```python
from build123d import *

# Parameters (mm, degrees)
AX_PCB_FLAT_FRONT_COMPARTMENT_START        = 25
SKETCH_1_W                                 = 90
SKETCH_1_H                                 = 130
SKETCH_1_R                                 = 1.75
AX_PCB_FLAT_FRONT_COMPARTMENT_DEPTH        = 1.6
J10_FRONT_CAMERA_HEADER_START              = 26.6
SKETCH_2_W                                 = 58.4
SKETCH_2_H                                 = 8.8
J10_FRONT_CAMERA_HEADER_DEPTH              = 8
J11_REAR_IDC40_START                       = 26.6
SKETCH_3_W                                 = 58.4
SKETCH_3_H                                 = 8.8
J11_REAR_IDC40_DEPTH                       = 8
HDMI_LEFT_START                            = 26.6
SKETCH_5_W                                 = 17
SKETCH_5_H                                 = 12
HDMI_LEFT_DEPTH                            = 8
USB_HOST_LEFT_START                        = 26.6
SKETCH_6_W                                 = 18
SKETCH_6_H                                 = 14
USB_HOST_LEFT_DEPTH                        = 12
RJ45_LEFT_START                            = 26.6
SKETCH_7_W                                 = 22
SKETCH_7_H                                 = 16
RJ45_LEFT_DEPTH                            = 14
DC5521_APPROX_BODY_CLEAR_CAMERA_EDGE_START = 26.6
SKETCH_8_W                                 = 12
SKETCH_8_H                                 = 12
DC5521_APPROX_BODY_CLEAR_CAMERA_EDGE_DEPTH = 12


with BuildPart() as part:
    # 草图1 → AX_PCB_flat_front_compartment (new body)
    with BuildSketch(Plane.XY.offset(AX_PCB_FLAT_FRONT_COMPARTMENT_START)):
        with Locations((0, -77)):
            Rectangle(SKETCH_1_W, SKETCH_1_H)
        with Locations((-41, -138)):
            Circle(SKETCH_1_R, mode=Mode.SUBTRACT)
        with Locations((41, -138)):
            Circle(SKETCH_1_R, mode=Mode.SUBTRACT)
        with Locations((41, -16)):
            Circle(SKETCH_1_R, mode=Mode.SUBTRACT)
        with Locations((-41, -16)):
            Circle(SKETCH_1_R, mode=Mode.SUBTRACT)
    extrude(amount=AX_PCB_FLAT_FRONT_COMPARTMENT_DEPTH)

    # 草图2 → J10_front_camera_header (add)
    with BuildSketch(Plane.XY.offset(J10_FRONT_CAMERA_HEADER_START)):
        with Locations((0, -137.5)):
            Rectangle(SKETCH_2_W, SKETCH_2_H)
    extrude(amount=J10_FRONT_CAMERA_HEADER_DEPTH)

    # 草图3 → J11_rear_IDC40 (add)
    with BuildSketch(Plane.XY.offset(J11_REAR_IDC40_START)):
        with Locations((0, -16.5)):
            Rectangle(SKETCH_3_W, SKETCH_3_H)
    extrude(amount=J11_REAR_IDC40_DEPTH)

    # 草图5 → HDMI_left (add)
    with BuildSketch(Plane.XY.offset(HDMI_LEFT_START)):
        with Locations((-39.5, -37)):
            Rectangle(SKETCH_5_W, SKETCH_5_H)
    extrude(amount=HDMI_LEFT_DEPTH)

    # 草图6 → USB_HOST_left (add)
    with BuildSketch(Plane.XY.offset(USB_HOST_LEFT_START)):
        with Locations((-39, -97)):
            Rectangle(SKETCH_6_W, SKETCH_6_H)
    extrude(amount=USB_HOST_LEFT_DEPTH)

    # 草图7 → RJ45_left (add)
    with BuildSketch(Plane.XY.offset(RJ45_LEFT_START)):
        with Locations((-37, -60)):
            Rectangle(SKETCH_7_W, SKETCH_7_H)
    extrude(amount=RJ45_LEFT_DEPTH)

    # 草图8 → DC5521_approx_body_clear_camera_edge (add)
    with BuildSketch(Plane.XY.offset(DC5521_APPROX_BODY_CLEAR_CAMERA_EDGE_START)):
        with Locations((-42, -128)):
            Rectangle(SKETCH_8_W, SKETCH_8_H)
    extrude(amount=DC5521_APPROX_BODY_CLEAR_CAMERA_EDGE_DEPTH)


solid = part.part
```
Verification items for the finished model (mm, model axes). A direction names the side the tool comes from. Coordinates: 2 decimals unless noted, no trailing zeros. Write each loop counter-clockwise with the first axis right and the second up, starting at its lowest first coordinate (ties: lowest second). Pieces come first, ordered by that corner, then holes. Notation, with made-up numbers: M 32,45 L 62,45 A32 ccw 62,79 Z; hole C -6.75,41 d4. An arc over 180 degrees is marked long. One line per item, written item: value.
Item 1: Mould release check, pull along X, two halves, no side actions. Record for faces 1 (the flat face through (-48, -128, 33)), 2 (the flat face through (0, -12.1, 31)), 3 (the cylindrical face through (-40.19, -139.55, 25.79)), 4 (the flat face through (29.2, -138, 31)): pulls with the +X half, pulls with the -X half, needs draft (parallel to the pull), parting line crosses it, or undercut.
Check sheet entries:
face 1: pulls with the -X half
face 2: needs draft
face 3: undercut
face 4: pulls with the +X half
Item 2: Section check D-D, the plane y = -129.5. Record the boundary of the cut face in (x, z), plus the area to 3 significant figures.
Check sheet entries:
outline: M -48,26.6 L -45,26.6 L -45,25 L 45,25 L 45,26.6 L -36,26.6 L -36,38.6 L -48,38.6 Z
area: 288 mm^2
Item 3: Section check C-C, the plane z = 31.75. Record the boundary of the cut face in (x, y).
Check sheet entries:
outline: M -48,-134 L -36,-134 L -36,-122 L -48,-122 Z; M -48,-104 L -30,-104 L -30,-90 L -48,-90 Z; M -48,-68 L -26,-68 L -26,-52 L -48,-52 Z; M -48,-43 L -31,-43 L -31,-31 L -48,-31 Z; M -29.2,-141.9 L 29.2,-141.9 L 29.2,-133.1 L -29.2,-133.1 Z; M -29.2,-20.9 L 29.2,-20.9 L 29.2,-12.1 L -29.2,-12.1 Z
Item 4: Scan lines: line 1 along X through (y, z) = (-138, 25.9); line 2 along Y through (x, z) = (41, 25.4); line 3 along Y through (x, z) = (-39, 36.5). Record each from-to range of solid material in increasing order.
Check sheet entries:
line 1: x = -45 to -42.75, -39.25 to 39.25, 42.75 to 45
line 2: y = -142 to -139.75, -136.25 to -17.75, -14.25 to -12
line 3: y = -134 to -122, -104 to -90, -68 to -52
Item 5: Access from +Z, -Z, +X, -X, +Y, -Y to the whole of each face (thin tool, end or side, straight path). Record for faces 5 (the flat face through (-29.2, -17, 31)), 6 (the flat face through (-47, -60, 26.6)), 7 (the flat face through (-40, -37, 34.6)).
Check sheet entries:
face 5: +Z, -X, +Y
face 6: -Z, -X, +Y, -Y
face 7: +Z, +X, -X, +Y
Item 6: Section check B-B, the plane x = -41. Record the boundary of the cut face in (y, z), plus the area to 3 significant figures.
Check sheet entries:
outline: M -142,25 L -139.75,25 L -139.75,26.6 L -142,26.6 Z; M -136.25,25 L -17.75,25 L -17.75,26.6 L -31,26.6 L -31,34.6 L -43,34.6 L -43,26.6 L -52,26.6 L -52,40.6 L -68,40.6 L -68,26.6 L -90,26.6 L -90,38.6 L -104,38.6 L -104,26.6 L -122,26.6 L -122,38.6 L -134,38.6 L -134,26.6 L -136.25,26.6 Z; M -14.25,25 L -12,25 L -12,26.6 L -14.25,26.6 Z
area: 829 mm^2
Item 7: Section check A-A, the plane y = -16. Record the boundary of the cut face in (x, z).
Check sheet entries:
outline: M -45,25 L -42.75,25 L -42.75,26.6 L -45,26.6 Z; M -39.25,25 L 39.25,25 L 39.25,26.6 L 29.2,26.6 L 29.2,34.6 L -29.2,34.6 L -29.2,26.6 L -39.25,26.6 Z; M 42.75,25 L 45,25 L 45,26.6 L 42.75,26.6 Z
Item 8: Gauge pin test, flat ends, axial feed: pin 1 Ø5.5 at (x, y) = (41, -138) entering from +Z; pin 2 Ø11 at (x, y) = (-35.5, -98.5) entering from +Z; pin 3 Ø3.5 at (y, z) = (-126, 35.5) entering from +X; pin 4 Ø3 at (x, y) = (-41, -138) entering from +Z. Record the tip position at first contact, or that the pin passes through.
Check sheet entries:
pin 1: stops at z = 26.6
pin 2: stops at z = 38.6
pin 3: stops at x = -36
pin 4: passes through
